Geometry check sheet. Reference: drawing and pictorial views, mm from the part's lowest x, y, z. A direction names the side the tool comes from. Round coordinates to 2 decimals unless told otherwise and drop trailing zeros. Write each loop counter-clockwise with the first axis right and the second up, starting at its lowest first coordinate (ties: lowest second). Pieces come first, ordered by that corner, then holes. Notation, with made-up numbers: (85, 29) - (112, 29) arc R21 ccw to (112, 36) - close; hole circle Ø2 at (39.25, 85). An arc over 180 degrees is marked (long way). Use one line per item in the form item = value. Start each with the question number.
1) Section check C-C (y = 30.5). Record the boundary of the cut face in (x, z).
2) Draft check along Z on the marked faces 1, 2 and 3. Enter one of: +Z half, -Z half, draft (parallel to the pull), parting line (faces both ways), or undercut.
3) Set-up check for the marked faces 4, 5, 6, 7 and 8: record each of +Z, -Z, +X, -X, +Y, -Y from which the full face is reachable in a straight line by a thin tool's end or side.
4) Section check A-A (z = 12.5). Record the boundary of the cut face in (x, y).
5) Section check B-B (x = 36). Record the boundary of the cut face in (y, z), then the cut area to 3 significant figures.
6) Section check D-D (x = 8). Record the boundary of the cut face in (y, z).
7) Gauge pin test, flat ends, axial feed: P1, Ø17.5, axis at x = 31, z = 26, coming from the +Y side; P2, Ø10.5, axis at y = 8.5, z = 30.5, coming from the -X side; P3, Ø10, axis at y = 29.5, z = 23, coming from the -X side; P4, Ø5, axis at x = 18, z = 5.5, coming from the +Y side. Record the tip position at first contact, or that the pin passes through.
8) Scan lines: probe 1 along Y at (x, z) = (35.5, 9.5); probe 2 along X at (y, z) = (26, 23.5); probe 3 along X at (y, z) = (3.5, 32.5). Record each from-to range of solid material in increasing order.
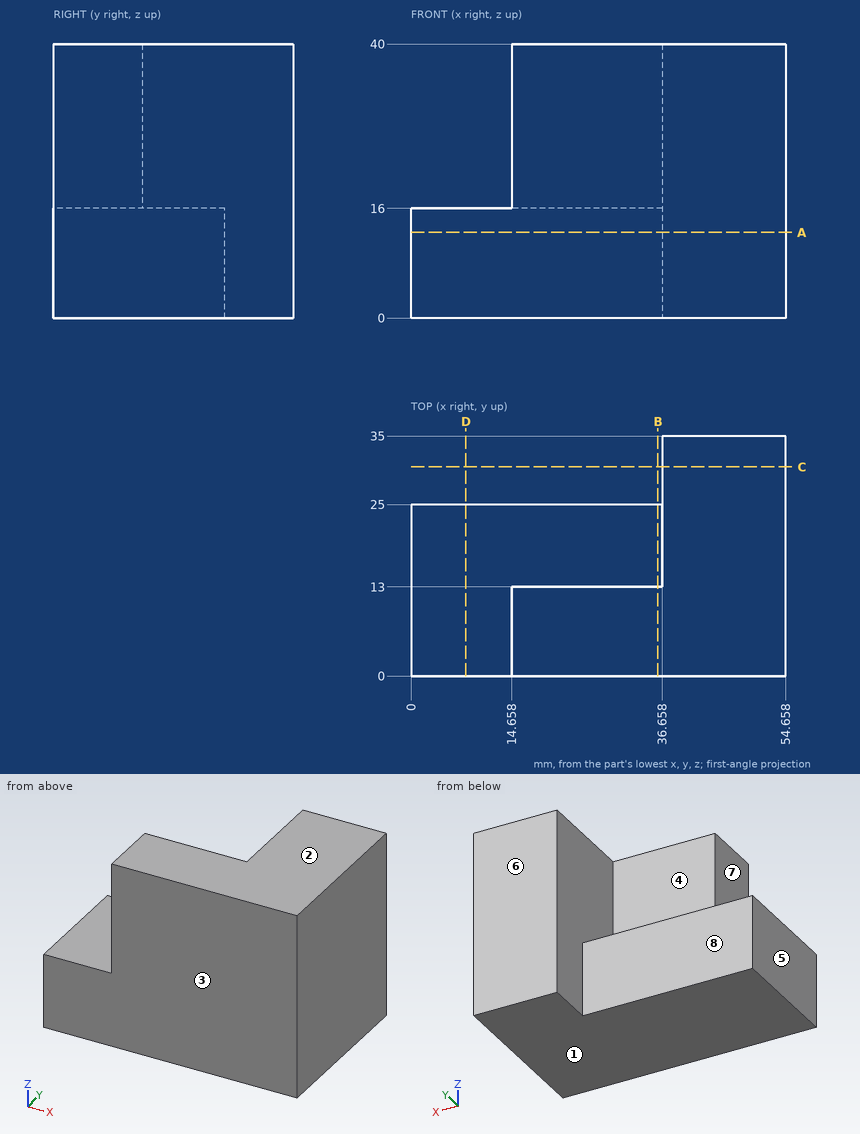
Results are:
q1.outline = (36.66, 0) - (54.66, 0) - (54.66, 40) - (36.66, 40) - close
q2.face_1 = -Z half
q2.face_2 = +Z half
q2.face_3 = draft
q3.face_4 = +Z, -X, +Y
q3.face_5 = +Z, -Z, -X, +Y, -Y
q3.face_6 = +Z, -Z, +X, -X, +Y
q3.face_7 = +Z, -X, +Y, -Y
q3.face_8 = +Z, -Z, -X, +Y
q4.outline = (0, 0) - (54.66, 0) - (54.66, 35) - (36.66, 35) - (36.66, 25) - (0, 25) - close
q5.outline = (0, 0) - (25, 0) - (25, 16) - (13, 16) - (13, 40) - (0, 40) - close
q5.area = 712 mm²
q6.outline = (0, 0) - (25, 0) - (25, 16) - (0, 16) - close
q7.P1 = 35
q7.P2 = 14.66
q7.P3 = 36.66
q7.P4 = 25
q8.probe_1 = 0 to 25
q8.probe_2 = 36.66 to 54.66
q8.probe_3 = 14.66 to 54.66
